```python
from build123d import *

# Parameters (mm, degrees)
SKETCH_1_R      = 1.4
SKETCH_1_W      = 12.8
SKETCH_1_H      = 6
EXTRUDE_1_DEPTH = 6


with BuildPart() as part:
    # Эскиз1 → Бобышка-Вытянуть1 (new body)
    with BuildSketch(Plane.XY):
        with BuildLine():
            Line((-167.182566644, 6), (64.127433356, 6))
            ThreePointArc((64.127433356, 6), (74.734035074, 10.393398282), (79.127433356, 21))
            Line((79.127433356, 21), (79.127433356, 44))
            Line((79.127433356, 44), (79.127433356, 52))
            ThreePointArc((79.127433356, 52), (80.59189945, 55.535533906), (84.127433356, 57))
            Line((84.127433356, 57), (91.127433356, 57))
            Line((91.127433356, 57), (91.127433356, 49))
            Line((91.127433356, 49), (91.127433356, 6))
            Line((91.127433356, 6), (91.127433356, -11))
            Line((91.127433356, -11), (-162.182566644, -11))
            Line((-162.182566644, -11), (-167.182566644, -6))
            Line((-167.182566644, -6), (-167.182566644, 6))
        make_face()
        with Locations((87.177433356, 0)):
            Circle(SKETCH_1_R, mode=Mode.SUBTRACT)
        with Locations((87.177433356, 44)):
            Circle(SKETCH_1_R, mode=Mode.SUBTRACT)
        with Locations((44.817433356, 0)):
            Rectangle(SKETCH_1_W, SKETCH_1_H, mode=Mode.SUBTRACT)
        with Locations((-45.982566644, 0)):
            Rectangle(SKETCH_1_W, SKETCH_1_H, mode=Mode.SUBTRACT)
        with Locations((-146.782566644, 0)):
            Rectangle(SKETCH_1_W, SKETCH_1_H, mode=Mode.SUBTRACT)
    extrude(amount=EXTRUDE_1_DEPTH)


solid = part.part
```
Verification items for the finished model (mm, model axes). A direction names the side the tool comes from. Give positions to 0.01 mm unless a question says otherwise; leave off trailing zeros. Order: outer loops, then holes, each group sorted by start corner. A loop starts at its lowest first (then second) coordinate and runs counter-clockwise, first axis right, second up. Notation, with made-up numbers: (-22, 81.25) -> (-11, 81.25) arc R17 cw to (-11, 112.25) -> close; hole circle Ø9 at (45, 23.5). An arc over 180 degrees is marked (long way). Use a Markdown table: item, result.
1) Section check A-A, the plane x = 43. Record the boundary of the cut face in (y, z), then the cut area to 3 significant figures.
Results:
| item | result |
|---|---|
| outline | (-11, 0) -> (-3, 0) -> (-3, 6) -> (-11, 6) -> close; (3, 0) -> (6, 0) -> (6, 6) -> (3, 6) -> close |
| area | 66.0 mm² |
2) Material ranges on probe 1 along Y at (x, z) = (-44, 3.3); probe 2 along X at (y, z) = (20, 0.95); probe 3 along Y at (x, z) = (4.5, 4.25), recorded low to high.
Results:
| item | result |
|---|---|
| probe 1 | -11 to -3, 3 to 6 |
| probe 2 | 79.09 to 91.13 |
| probe 3 | -11 to 6 |
3) Depth check by flat-ended pin: pin 1 Ø3 at (x, z) = (-88, 2) entering from +Y; pin 2 Ø1.5 at (y, z) = (40, 4) entering from -X. Enter the tip coordinate at first touch or a pass-through.
Results:
| item | result |
|---|---|
| pin 1 | y = 6 |
| pin 2 | x = 79.13 |
4) Section check B-B, the plane z = 2.55. Record the boundary of the cut face in (x, y), then the cut area to 3 significant figures.
Results:
| item | result |
|---|---|
| outline | (-167.18, -6) -> (-162.18, -11) -> (91.13, -11) -> (91.13, 57) -> (84.13, 57) arc R5 ccw to (79.13, 52) -> (79.13, 21) arc R15 cw to (64.13, 6) -> (-167.18, 6) -> close; hole (-153.18, -3) -> (-140.38, -3) -> (-140.38, 3) -> (-153.18, 3) -> close; hole (-52.38, -3) -> (-39.58, -3) -> (-39.58, 3) -> (-52.38, 3) -> close; hole (38.42, -3) -> (51.22, -3) -> (51.22, 3) -> (38.42, 3) -> close; hole circle Ø2.8 at (87.18, 0); hole circle Ø2.8 at (87.18, 44) |
| area | 4,790 mm² |
5) Mould release check, pull along Y, two halves, no side actions. Record for faces 4 (the flat face through (-167.183, 0, 3)), 5 (the cylindrical face through (80.553, 55.496, 2.958)), 6 (the flat face through (-52.383, 0, 3)): pulls with the +Y half, pulls with the -Y half, needs draft (parallel to the pull), parting line crosses it, or undercut.
Results:
| item | result |
|---|---|
| face 4 | needs draft |
| face 5 | pulls with the +Y half |
| face 6 | undercut |
6) Tool access check on faces 1 (the flat face through (-28, 0, 0)), 2 (the flat face through (-53, 6, 3)), 3 (the flat face through (45, -3, 3)). Record the directions out of +Z, -Z, +X, -X, +Y, -Y that give a thin tool (end or side, any length) a straight path to the whole face; none if there is none.
Results:
| item | result |
|---|---|
| face 1 | -Z, +X, -X, +Y, -Y |
| face 2 | +Z, -Z, -X, +Y |
| face 3 | +Z, -Z |
